from build123d import *

# Parameters (mm, degrees)
SKETCH1_R             = 3.75
SKETCH1_R_2           = 1.6
BOSS_EXTRUDE3_DEPTH   = 3
BOSS_EXTRUDE3_2_DEPTH = 3
BOSS_EXTRUDE3_3_DEPTH = 3
BOSS_EXTRUDE3_4_DEPTH = 3
BOSS_EXTRUDE4_DEPTH   = 65
SKETCH3_R             = 55
SKETCH3_R_2           = 45
SKETCH3_R_3           = 1.6
BOSS_EXTRUDE5_DEPTH   = 5


with BuildPart() as part:
    # Sketch1 → Boss-Extrude3 (new body)
    with BuildSketch(Plane(origin=(0, 0, 0), x_dir=(1, 0, 0), z_dir=(0, 1, 0))):
        with Locations((13.5, 43)):
            Circle(SKETCH1_R)
        with Locations((13.5, 43)):
            Circle(SKETCH1_R_2, mode=Mode.SUBTRACT)
    extrude(amount=BOSS_EXTRUDE3_DEPTH)



with BuildPart() as body_2:
    # Sketch1 → Boss-Extrude3 2 (new body)
    with BuildSketch(Plane(origin=(0, 0, 0), x_dir=(1, 0, 0), z_dir=(0, 1, 0))):
        with Locations((-13.5, 43)):
            Circle(SKETCH1_R)
        with Locations((-13.5, 43)):
            Circle(SKETCH1_R_2, mode=Mode.SUBTRACT)
    extrude(amount=BOSS_EXTRUDE3_2_DEPTH)


with BuildPart() as body_3:
    # Sketch1 → Boss-Extrude3 3 (new body)
    with BuildSketch(Plane(origin=(0, 0, 0), x_dir=(1, 0, 0), z_dir=(0, 1, 0))):
        with Locations((-13.5, -43)):
            Circle(SKETCH1_R)
        with Locations((-13.5, -43)):
            Circle(SKETCH1_R_2, mode=Mode.SUBTRACT)
    extrude(amount=BOSS_EXTRUDE3_3_DEPTH)


with BuildPart() as body_4:
    # Sketch1 → Boss-Extrude3 4 (new body)
    with BuildSketch(Plane(origin=(0, 0, 0), x_dir=(1, 0, 0), z_dir=(0, 1, 0))):
        with Locations((13.5, -43)):
            Circle(SKETCH1_R)
        with Locations((13.5, -43)):
            Circle(SKETCH1_R_2, mode=Mode.SUBTRACT)
    extrude(amount=BOSS_EXTRUDE3_4_DEPTH)


with BuildPart() as part_1:
    add(part.part)

    add(body_2.part)  # Boss-Extrude4 merges body 2

    add(body_3.part)  # Boss-Extrude4 merges body 3

    add(body_4.part)  # Boss-Extrude4 merges body 4
    # Sketch1_7 → Boss-Extrude4 (add)
    with BuildSketch(Plane(origin=(0, 0, 0), x_dir=(1, 0, 0), z_dir=(0, 1, 0))):
        with BuildLine():
            ThreePointArc((19.323265389, -40.640022327), (18.170769041, -41.168229892), (17.003850477, -41.663762059))
            ThreePointArc((17.003850477, -41.663762059), (17.187949246, -42.320639746), (17.25, -43))
            ThreePointArc((17.25, -43), (13.956514354, -46.722108897), (9.861149523, -43.906237941))
            ThreePointArc((9.861149523, -43.906237941), (8.620399067, -44.166601861), (7.372806564, -44.391910562))
            Line((7.372806564, -44.391910562), (9.011208023, -54.256779576))
            ThreePointArc((9.011208023, -54.256779576), (16.474595828, -52.474638563), (23.617324364, -49.671138399))
            Line((23.617324364, -49.671138399), (19.323265389, -40.640022327))
        make_face()
        with BuildLine():
            ThreePointArc((-9.861149523, -43.906237941), (-14.623267897, -46.577816266), (-17.003850477, -41.663762059))
            ThreePointArc((-17.003850477, -41.663762059), (-18.170769041, -41.168229892), (-19.323265389, -40.640022327))
            Line((-19.323265389, -40.640022327), (-23.617324364, -49.671138399))
            ThreePointArc((-23.617324364, -49.671138399), (-16.474595828, -52.474638563), (-9.011208023, -54.256779576))
            Line((-9.011208023, -54.256779576), (-7.372806564, -44.391910562))
            ThreePointArc((-7.372806564, -44.391910562), (-8.620399067, -44.166601861), (-9.861149523, -43.906237941))
        make_face()
        with BuildLine():
            ThreePointArc((17.003850477, 41.663762059), (18.170769041, 41.168229892), (19.323265389, 40.640022327))
            Line((19.323265389, 40.640022327), (23.617324364, 49.671138399))
            ThreePointArc((23.617324364, 49.671138399), (16.474595828, 52.474638563), (9.011208023, 54.256779576))
            Line((9.011208023, 54.256779576), (7.372806564, 44.391910562))
            ThreePointArc((7.372806564, 44.391910562), (8.620399067, 44.166601861), (9.861149523, 43.906237941))
            ThreePointArc((9.861149523, 43.906237941), (13.956514354, 46.722108897), (17.25, 43))
            ThreePointArc((17.25, 43), (17.187949246, 42.320639746), (17.003850477, 41.663762059))
        make_face()
        with BuildLine():
            Line((-23.617324364, 49.671138399), (-19.323265389, 40.640022327))
            ThreePointArc((-19.323265389, 40.640022327), (-18.170769041, 41.168229892), (-17.003850477, 41.663762059))
            ThreePointArc((-17.003850477, 41.663762059), (-14.623267897, 46.577816266), (-9.861149523, 43.906237941))
            ThreePointArc((-9.861149523, 43.906237941), (-8.620399067, 44.166601861), (-7.372806564, 44.391910562))
            Line((-7.372806564, 44.391910562), (-9.011208023, 54.256779576))
            ThreePointArc((-9.011208023, 54.256779576), (-16.474595828, 52.474638563), (-23.617324364, 49.671138399))
        make_face()
    extrude(amount=BOSS_EXTRUDE4_DEPTH)

    # Sketch3 → Boss-Extrude5 (add)
    with BuildSketch(Plane(origin=(0, 65, 0), x_dir=(1, 0, 0), z_dir=(0, 1, 0))):
        Circle(SKETCH3_R)
        Circle(SKETCH3_R_2, mode=Mode.SUBTRACT)
        with Locations((0, 50)):
            Circle(SKETCH3_R_3, mode=Mode.SUBTRACT)
        with Locations((25, 43.301270189)):
            Circle(SKETCH3_R_3, mode=Mode.SUBTRACT)
        with Locations((43.301270189, 25)):
            Circle(SKETCH3_R_3, mode=Mode.SUBTRACT)
        with Locations((50, 0)):
            Circle(SKETCH3_R_3, mode=Mode.SUBTRACT)
        with Locations((43.301270189, -25)):
            Circle(SKETCH3_R_3, mode=Mode.SUBTRACT)
        with Locations((25, -43.301270189)):
            Circle(SKETCH3_R_3, mode=Mode.SUBTRACT)
        with Locations((0, -50)):
            Circle(SKETCH3_R_3, mode=Mode.SUBTRACT)
        with Locations((-25, -43.301270189)):
            Circle(SKETCH3_R_3, mode=Mode.SUBTRACT)
        with Locations((-43.301270189, -25)):
            Circle(SKETCH3_R_3, mode=Mode.SUBTRACT)
        with Locations((-50, 0)):
            Circle(SKETCH3_R_3, mode=Mode.SUBTRACT)
        with Locations((-43.301270189, 25)):
            Circle(SKETCH3_R_3, mode=Mode.SUBTRACT)
        with Locations((-25, 43.301270189)):
            Circle(SKETCH3_R_3, mode=Mode.SUBTRACT)
    extrude(amount=BOSS_EXTRUDE5_DEPTH)


solid = part_1.part
Design review of the part built by this model. Coordinates are the model's own, in mm. A direction names the side the tool comes from. Coordinates: 2 decimals unless noted, no trailing zeros. Order: outer loops, then holes, each group sorted by start corner. A loop starts at its lowest first (then second) coordinate and runs counter-clockwise, first axis right, second up.
Item 1: Take a section at D-D, the plane x = 33. Write out the cut boundary in (y, z).
Item 2: The part is to be moulded in two halves that separate along Z. For faces 5 (the flat face through (8.18, 32.04, 49.26)), 6 (the flat face through (-16, 0, 47)), 7 (the cylindrical face through (51.526, 67.465, -0.481)), 8 (the cylindrical face through (-25.347, 67.465, 44.863)), say which applies: pulls with the +Z half, pulls with the -Z half, needs draft (parallel to the pull), parting line crosses it, or undercut.
Item 3: For pin 1 Ø8 at (x, z) = (15.5, 42) entering from +Y; pin 2 Ø4 at (x, z) = (-43.3, -25) entering from -Y; pin 3 Ø6 at (x, y) = (-13.5, 32) entering from -Z, all flat-tipped, find the tip position at first contact; note any pin that passes through.
Item 4: Take a section at A-A, the plane x = 0. Write out the cut boundary in (y, z).
Item 5: Take a section at B-B, the plane y = 39.5. Write out the cut boundary in (x, z).
Item 6: For line 1 (X direction, y = 67.4, z = 0); line 2 (Z direction, x = 25, y = 67.55); line 3 (X direction, y = 2, z = 43), list the stretches that pass through material, from the lowest coordinate up.
Item 7: Take a section at C-C, the plane z = 25. Write out the cut boundary in (x, y), then the cut area to 3 significant figures.
Item 8: For faces 1 (the flat face through (21.5, 32.04, 45.22)), 2 (the cylindrical face through (-14.77, 1.48, 43.97)), 3 (the flat face through (2, 65, -50)), 4 (the flat face through (13, 3, -41)), list the 3-axis set-ups (+Z, -Z, +X, -X, +Y, -Y) from which the entire face can be reached by the end or side of a thin tool; tool diameter is ignored.
The answers:
1. outline: (65, -44) - (70, -44) - (70, -30.59) - (65, -30.59) - close; (65, 30.59) - (70, 30.59) - (70, 44) - (65, 44) - close
2. face 5: pulls with the +Z half
2. face 6: needs draft
2. face 7: undercut
2. face 8: undercut
3. pin 1: stops at y = 70
3. pin 2: stops at y = 65
3. pin 3: stops at z = -53.99
4. outline: (65, -55) - (70, -55) - (70, -51.6) - (65, -51.6) - close; (65, -48.4) - (70, -48.4) - (70, -45) - (65, -45) - close; (65, 45) - (70, 45) - (70, 48.4) - (65, 48.4) - close; (65, 51.6) - (70, 51.6) - (70, 55) - (65, 55) - close
5. outline: (-23.62, -49.67) arc R55 ccw to (-9.01, -54.26) - (-7.37, -44.39) arc R45 cw to (-9.86, -43.91) arc R3.75 cw (long way) to (-17, -41.66) arc R45 cw to (-19.32, -40.64) - close; (-23.62, 49.67) - (-19.32, 40.64) arc R45 cw to (-17, 41.66) arc R3.75 cw (long way) to (-9.86, 43.91) arc R45 cw to (-7.37, 44.39) - (-9.01, 54.26) arc R55 ccw to start; (7.37, -44.39) - (9.01, -54.26) arc R55 ccw to (23.62, -49.67) - (19.32, -40.64) arc R45 cw to (17, -41.66) arc R3.75 cw (long way) to (9.86, -43.91) arc R45 cw to start; (7.37, 44.39) arc R45 cw to (9.86, 43.91) arc R3.75 cw (long way) to (17, 41.66) arc R45 cw to (19.32, 40.64) - (23.62, 49.67) arc R55 ccw to (9.01, 54.26) - close
6. line 1: x = -55 to -51.6, -48.4 to -45, 45 to 48.4, 51.6 to 55
6. line 2: z = -48.99 to -44.9, -41.7 to -37.42, 37.42 to 41.7, 44.9 to 48.99
6. line 3: x = -20.45 to -15.1, -11.9 to -9.75, 9.75 to 11.9, 15.1 to 20.45
7. outline: (-48.99, 65) - (-44.9, 65) - (-44.9, 70) - (-48.99, 70) - close; (-41.7, 65) - (-37.42, 65) - (-37.42, 70) - (-41.7, 70) - close; (37.42, 65) - (41.7, 65) - (41.7, 70) - (37.42, 70) - close; (44.9, 65) - (48.99, 65) - (48.99, 70) - (44.9, 70) - close
7. area: 83.7 mm2
8. face 1: +X, -Y
8. face 2: -Y
8. face 3: -Z, -Y
8. face 4: none
